Check sheet for the drawn part. Datum: minimum x, y, z corner. Units: mm. Round coordinates to 2 decimals unless told otherwise and drop trailing zeros. Loops run counter-clockwise (first coordinate to the right, second up) from the corner with the lowest first, then second, coordinate; pieces in that order, holes last.
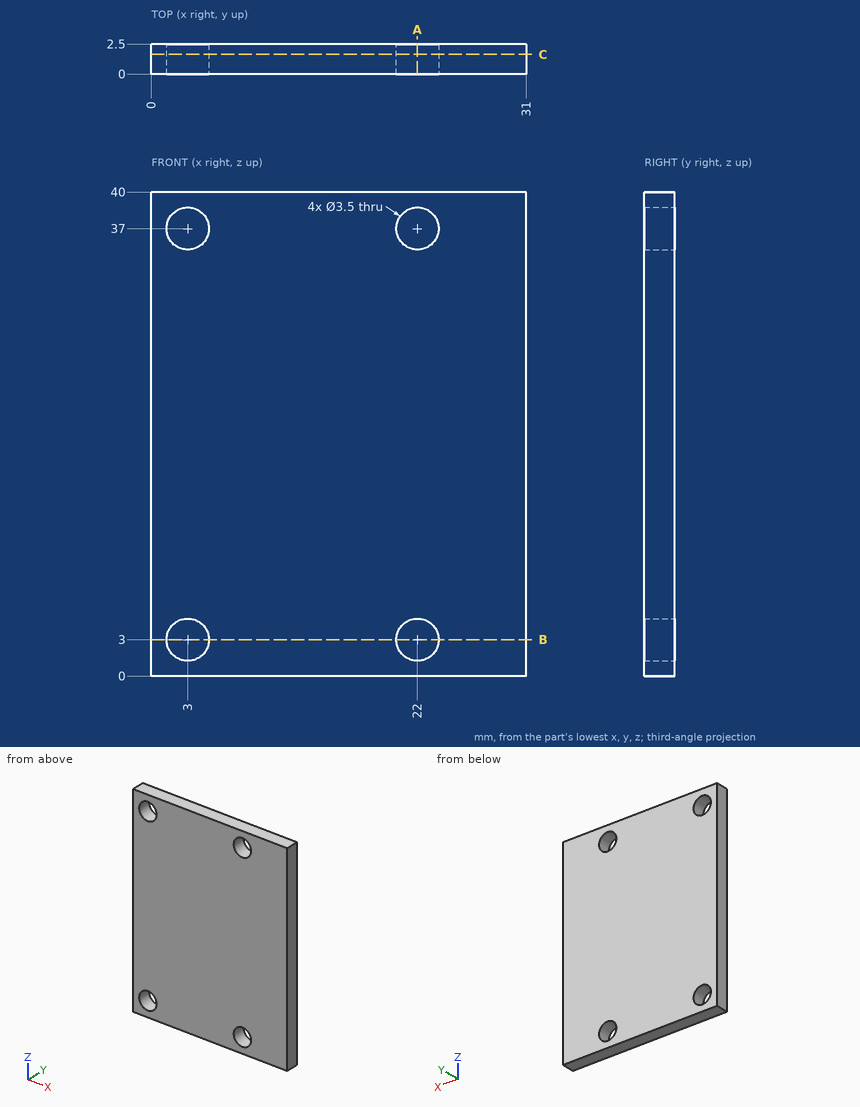
1. Gauge pin test, flat end, axial feed: P1, Ø3, axis at x = 15.5, z = 18, coming from the -Y side. Record the tip position at first contact, or that the pin passes through.
2. Section check B-B (z = 3). Enter the section's corners in (x, y).
3. Section check C-C (y = 1.65). Enter the section's corners in (x, z), then the cut area to 3 significant figures.
4. Scan lines: L1, parallel to Z at x = 3, y = 1.55; L2, parallel to X at y = 1.4, z = 3; L3, parallel to Z at x = 4.5, y = 0.4. Record each from-to range of solid material in increasing order.
5. Section check A-A (x = 22). Enter the section's corners in (y, z).
Taken from the geometry:
1. P1: stops at y = 0
2. outline: (0, 0) - (1.25, 0) - (1.25, 2.5) - (0, 2.5) - close; (4.75, 0) - (20.25, 0) - (20.25, 2.5) - (4.75, 2.5) - close; (23.75, 0) - (31, 0) - (31, 2.5) - (23.75, 2.5) - close
3. outline: (0, 0) - (31, 0) - (31, 40) - (0, 40) - close; hole circle Ø3.5 at (3, 3); hole circle Ø3.5 at (3, 37); hole circle Ø3.5 at (22, 3); hole circle Ø3.5 at (22, 37)
3. area: 1,200 mm2
4. L1: z = 0 to 1.25, 4.75 to 35.25, 38.75 to 40
4. L2: x = 0 to 1.25, 4.75 to 20.25, 23.75 to 31
4. L3: z = 0 to 2.1, 3.9 to 36.1, 37.9 to 40
5. outline: (0, 0) - (2.5, 0) - (2.5, 1.25) - (0, 1.25) - close; (0, 4.75) - (2.5, 4.75) - (2.5, 35.25) - (0, 35.25) - close; (0, 38.75) - (2.5, 38.75) - (2.5, 40) - (0, 40) - close
